Study the drawing (mm; zero at the part's minimum x, y, z) and answer. A direction names the side the tool comes from. Give positions to 0.01 mm unless a question says otherwise; leave off trailing zeros. Order: outer loops, then holes, each group sorted by start corner. A loop starts at its lowest first (then second) coordinate and runs counter-clockwise, first axis right, second up.
Item 1: Find the intervals of material crossed by line 1 along Z through (x, y) = (40, 33); line 2 along X through (y, z) = (54.5, 14.5); line 3 along Y through (x, z) = (52.5, 95.5), in increasing order.
Item 2: A cutting plane is placed at D-D (x = 25.5). Write down the section's boundary in (y, z).
Item 3: A cutting plane is placed at B-B (x = 40). Write down the section's boundary in (y, z), plus the area to 3 significant figures.
Item 4: Given pin 1 Ø10 at (y, z) = (33, 78) entering from +X; pin 2 Ø1.5 at (x, z) = (38, 81) entering from +Y; pin 3 Ø7.5 at (x, y) = (74.5, 16.5) entering from +Z, each flat-ended and moving along its own axis, determine where each tip first touches the part or whether it passes through.
Item 5: Which of the six approach directions +Z, -Z, +X, -X, +Y, -Y give full straight-line access (tool end or side, diameter ignored) to the marked faces 1, 2, 3 and 4?
Item 6: A cutting plane is placed at A-A (z = 132). Write down the section's boundary in (x, y).
Item 7: A cutting plane is placed at C-C (y = 46.5). Write down the section's boundary in (x, z).
Item 8: The mould has two halves that part along X. Classify the marked faces 5, 6, 7 and 8: +X half, -X half, draft (parallel to the pull), parting line (faces both ways), or undercut.
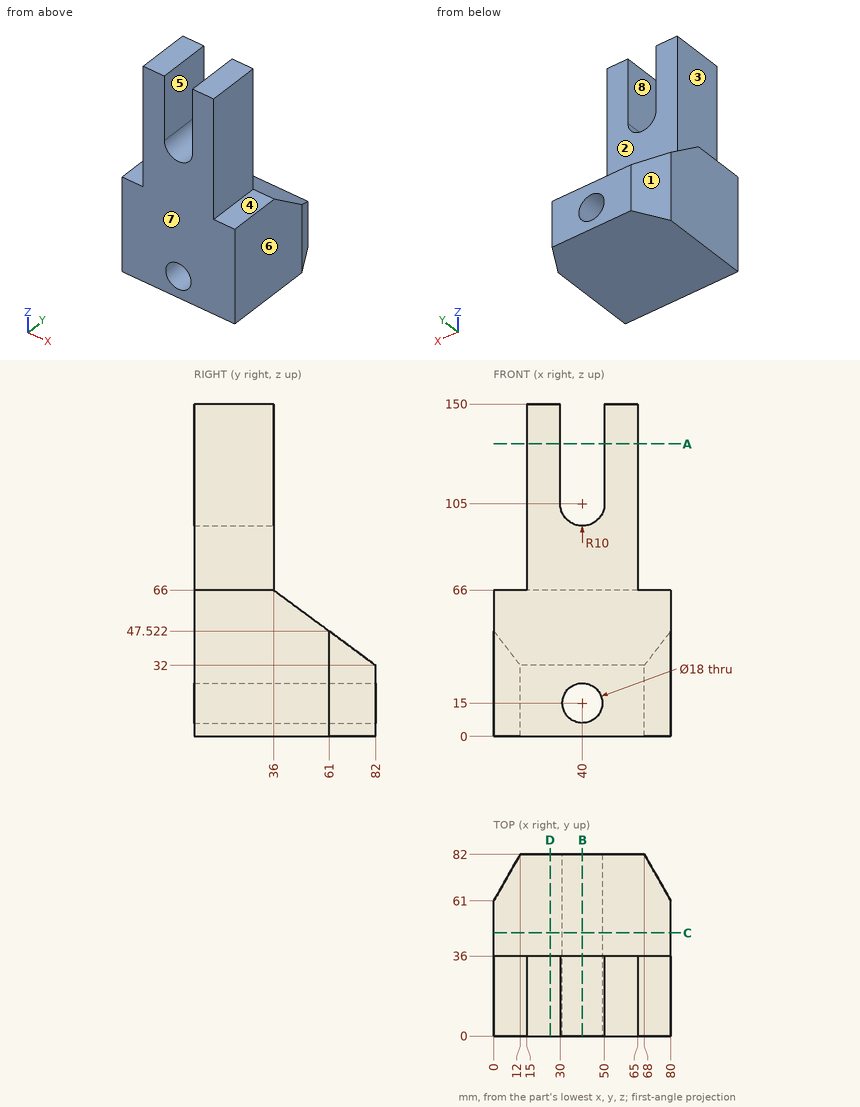
Response values:
1. line 1: z = 0 to 6, 24 to 95
1. line 2: x = 0 to 31.01, 48.99 to 80
1. line 3: y = 0 to 36
2. outline: (0, 0) - (82, 0) - (82, 32) - (36, 66) - (36, 150) - (0, 150) - close
3. outline: (0, 0) - (82, 0) - (82, 6) - (0, 6) - close; (0, 24) - (82, 24) - (82, 32) - (36, 66) - (36, 95) - (0, 95) - close
3. area: 4,200 mm2
4. pin 1: stops at x = 65
4. pin 2: stops at y = 36
4. pin 3: stops at z = 66
5. face 1: +Z, -Z, -X, +Y
5. face 2: +Z, +X, -X, +Y
5. face 3: +Z, -X, +Y, -Y
5. face 4: +Z, +X, +Y, -Y
6. outline: (15, 0) - (30, 0) - (30, 36) - (15, 36) - close; (50, 0) - (65, 0) - (65, 36) - (50, 36) - close
7. outline: (0, 0) - (80, 0) - (80, 58.24) - (0, 58.24) - close; hole circle Ø18 at (40, 15)
8. face 5: undercut
8. face 6: +X half
8. face 7: draft
8. face 8: undercut
